Source: CAD feature listing. Evaluate the final solid. Frame: model axes, mm. Face numbers are marked on the shaded views. Coordinates: 2 decimals unless noted, no trailing zeros. Loops run counter-clockwise (first coordinate to the right, second up) from the corner with the lowest first, then second, coordinate; pieces in that order, holes last. Notation, with made-up numbers: M 75.5,-3 L 108.5,-3 A31 cw 108.5,30 Z; hole C -30.75,17 d9. An arc over 180 degrees is marked long. One line per question, with ' | ' between items. Start each with the question number.
1. Section query C-C, the plane y = 14. State how many separate pieces and enclosed holes the cut face has, and give its area (3 significant figures).
2. Section query B-B, the plane z = 0. Output: boundary loops of the cut face in (x, y) (3 decimals), and give its area (3 significant figures).
3. Pin query (flat end, axial travel): P1, Ø5, axis at x = -11.11, z = 15.97, coming from the +Y side; P2, Ø3, axis at x = -8, y = 25.5, coming from the +Z side; P3, Ø3, axis at x = 20, y = 44.5, coming from the +Z side; P4, Ø8.5, axis at x = 8, y = 20, coming from the -Z side. Return the tip coordinate at first contact, or that it passes through.
4. Ray query, probe 1 along X at (y, z) = (29, -12.5); probe 2 along X at (y, z) = (35, -8); probe 3 along X at (y, z) = (7, -2) (3 decimals). Return the intervals inside material, ascending.
5. Mould query, pull axis X, two halves, no side actions, for the marked faces 1, 2 and 3. Classes: pulls with the +X half, pulls with the -X half, needs draft (parallel to the pull), parting line crosses it, or undercut.
6. Section query A-A, the plane x = 6. Output: boundary loops of the cut face in (y, z).
```python
from build123d import *

# Parameters (mm, degrees)
SKETCH1_R           = 25.6
BOSS_EXTRUDE1_DEPTH = 50.8
CHAMFER1_SIZE       = 0.2


with BuildPart() as part:
    # Sketch1 → Boss-Extrude1 (new body)
    with BuildSketch(Plane(origin=(0, 0, 0), x_dir=(1, 0, 0), z_dir=(0, 1, 0))):
        with Locations(Location((0, 0, 0), (0, 0, 270))):
            Circle(SKETCH1_R)
        with BuildLine():
            Line((0.445926966, 14.307233146), (9.721207865, 18.828932584))
            ThreePointArc((9.721207865, 18.828932584), (14.206192046, 16.688928934), (11.1125, 12.8))
            Line((11.1125, 12.8), (0.79375, 12.8))
            ThreePointArc((0.79375, 12.8), (0.020326988, 13.415267767), (0.445926966, 14.307233146))
        make_face(mode=Mode.SUBTRACT)
        with BuildLine():
            Line((8.770343138, 11.312685463), (18.931991258, 9.518943829))
            ThreePointArc((18.931991258, 9.518943829), (21.302557095, 5.151436949), (16.513852579, 3.823653912))
            Line((16.513852579, 3.823653912), (8.165808469, 9.888862984))
            ThreePointArc((8.165808469, 9.888862984), (7.901741428, 10.841231703), (8.770343138, 11.312685463))
        make_face(mode=Mode.SUBTRACT)
        with BuildLine():
            Line((13.744786325, 3.997076438), (20.911397465, -3.426957932))
            ThreePointArc((20.911397465, -3.426957932), (20.26206938, -8.353728859), (15.607474759, -6.613198009))
            Line((15.607474759, -6.613198009), (12.418805648, 3.200516418))
            ThreePointArc((12.418805648, 3.200516418), (12.764959212, 4.126213609), (13.744786325, 3.997076438))
        make_face(mode=Mode.SUBTRACT)
        with BuildLine():
            Line((13.469188303, -4.845279932), (14.903360593, -15.063878241))
            ThreePointArc((14.903360593, -15.063878241), (11.482159845, -18.668054176), (8.739572059, -14.524033065))
            Line((8.739572059, -14.524033065), (11.928241169, -4.710318638))
            ThreePointArc((11.928241169, -4.710318638), (12.752396442, -4.164877839), (13.469188303, -4.845279932))
        make_face(mode=Mode.SUBTRACT)
        with BuildLine():
            Line((8.04881815, -11.836904052), (3.202746521, -20.946909064))
            ThreePointArc((3.202746521, -20.946909064), (-1.683544487, -21.851817301), (-1.466550121, -16.887181144))
            Line((-1.466550121, -16.887181144), (6.88149399, -10.821972072))
            ThreePointArc((6.88149399, -10.821972072), (7.86885167, -10.865127511), (8.04881815, -11.836904052))
        make_face(mode=Mode.SUBTRACT)
        with BuildLine():
            Line((-0.445926966, -14.307233146), (-9.721207865, -18.828932584))
            ThreePointArc((-9.721207865, -18.828932584), (-14.206192046, -16.688928934), (-11.1125, -12.8))
            Line((-11.1125, -12.8), (-0.79375, -12.8))
            ThreePointArc((-0.79375, -12.8), (-0.020326988, -13.415267767), (-0.445926966, -14.307233146))
        make_face(mode=Mode.SUBTRACT)
        with BuildLine():
            Line((-8.770343138, -11.312685463), (-18.931991258, -9.518943829))
            ThreePointArc((-18.931991258, -9.518943829), (-21.302557095, -5.151436949), (-16.513852579, -3.823653912))
            Line((-16.513852579, -3.823653912), (-8.165808469, -9.888862984))
            ThreePointArc((-8.165808469, -9.888862984), (-7.901741428, -10.841231703), (-8.770343138, -11.312685463))
        make_face(mode=Mode.SUBTRACT)
        with BuildLine():
            Line((-13.744786325, -3.997076438), (-20.911397465, 3.426957932))
            ThreePointArc((-20.911397465, 3.426957932), (-20.26206938, 8.353728859), (-15.607474759, 6.613198009))
            Line((-15.607474759, 6.613198009), (-12.418805648, -3.200516418))
            ThreePointArc((-12.418805648, -3.200516418), (-12.764959212, -4.126213609), (-13.744786325, -3.997076438))
        make_face(mode=Mode.SUBTRACT)
        with BuildLine():
            Line((-13.469188303, 4.845279932), (-14.903360593, 15.063878241))
            ThreePointArc((-14.903360593, 15.063878241), (-11.482159845, 18.668054176), (-8.739572059, 14.524033065))
            Line((-8.739572059, 14.524033065), (-11.928241169, 4.710318638))
            ThreePointArc((-11.928241169, 4.710318638), (-12.752396442, 4.164877839), (-13.469188303, 4.845279932))
        make_face(mode=Mode.SUBTRACT)
        with BuildLine():
            Line((-8.04881815, 11.836904052), (-3.202746521, 20.946909064))
            ThreePointArc((-3.202746521, 20.946909064), (1.683544487, 21.851817301), (1.466550121, 16.887181144))
            Line((1.466550121, 16.887181144), (-6.88149399, 10.821972072))
            ThreePointArc((-6.88149399, 10.821972072), (-7.86885167, 10.865127511), (-8.04881815, 11.836904052))
        make_face(mode=Mode.SUBTRACT)
        Polygon((0, 10.998522628), (-9.525, 5.499261314), (-9.525, -5.499261314), (0, -10.998522628), (9.525, -5.499261314), (9.525, 5.499261314), align=None, mode=Mode.SUBTRACT)
    extrude(amount=BOSS_EXTRUDE1_DEPTH)

    # Chamfer1
    chamfer1_edges = [part.edges().sort_by_distance(p)[0] for p in [
        (-4.7625, 0, -8.248891971),
        (-9.525, 0, 0),
        (-4.7625, 0, 8.248891971),
        (4.7625, 0, 8.248891971),
        (9.525, 0, 0),
        (4.7625, 0, -8.248891971),
    ]]
    chamfer(chamfer1_edges, length=CHAMFER1_SIZE)


solid = part.part
```
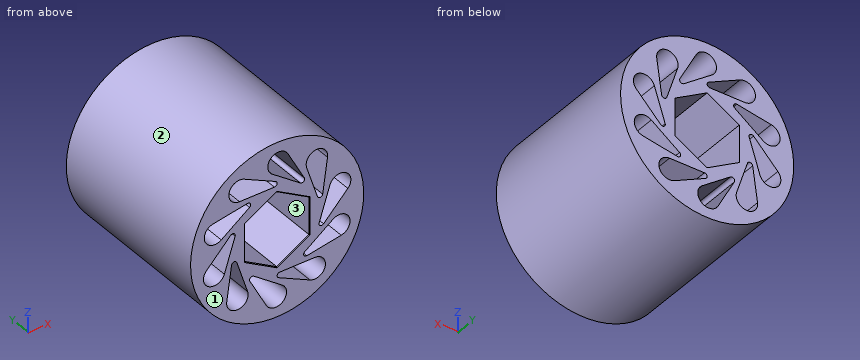
Taken from the geometry:
1) separate pieces: 1 | enclosed holes: 11 | area: 1,150 mm^2
2) outline: M -25.6,0 L -17.603,0 L -17.603,50.8 L -25.6,50.8 Z; M -13.459,0 L -9.725,0 L -9.525,0.2 L -9.525,50.8 L -13.459,50.8 Z; M 9.525,0.2 L 9.725,0 L 13.459,0 L 13.459,50.8 L 9.525,50.8 Z; M 17.603,0 L 25.6,0 L 25.6,50.8 L 17.603,50.8 Z | area: 1,210 mm^2
3) P1: through | P2: z = 24.76 | P3: z = 17.69 | P4: z = -25.32
4) probe 1: -22.34 to -14.54, -9.4 to -7.7, -4.57 to 22.34 | probe 2: -24.32 to -20.74, -16.51 to -13.91, -10.86 to -5.19, 5.19 to 10.77, 21.12 to 24.32 | probe 3: -25.522 to -19.534, -14.109 to -9.525, 9.525 to 12.809, 15.673 to 25.522
5) face 1: needs draft | face 2: parting line crosses it | face 3: undercut
6) outline: M 0,-24.89 L 50.8,-24.89 L 50.8,-17.01 L 0,-17.01 Z; M 0,-12.8 L 50.8,-12.8 L 50.8,-7.53 L 0.2,-7.53 L 0,-7.77 Z; M 0,7.77 L 0.2,7.53 L 50.8,7.53 L 50.8,11.46 L 0,11.46 Z; M 0,15.69 L 50.8,15.69 L 50.8,24.89 L 0,24.89 Z
